Could you check a few things on this drawing? It's one solid part, dimensions in mm from its lowest x, y, z. A direction names the side the tool comes from. Give positions to 0.01 mm unless a question says otherwise; leave off trailing zeros. Loops run counter-clockwise (first coordinate to the right, second up) from the corner with the lowest first, then second, coordinate; pieces in that order, holes last. Notation, with made-up numbers: M 27,75.25 L 79,75.25 A14 ccw 79,94.25 Z; hole C 1.25,46 d7. An arc over 180 degrees is marked long. Answer as CSV lines item,"result". Start each with the question number.
Item 1: For the marked faces 1 and 2, which set-ups out of +Z, -Z, +X, -X, +Y, -Y let a thin tool reach every point of the face, with its end or its side?
Item 2: If I drill on line 1 along Z through (x, y) = (0.95, 52); line 2 along Y through (x, z) = (0.9, 37.4); line 3 along Z through (x, y) = (1.1, 41.5), over which ranges is the centre line in solid material (lowest first)? Write a range as from..to.
Item 3: I want a section at D-D on y = 2.8. List the corners of the cut face in (x, z) for me, plus the area to 3 significant figures.
Item 4: I want a section at B-B on z = 37.4. List the corners of the cut face in (x, y) for me, plus the area to 3 significant figures.
Item 5: I want a section at A-A on y = 30.1. List the corners of the cut face in (x, z) for me, plus the area to 3 significant figures.
Item 6: I want a section at C-C on y = 56. List the corners of the cut face in (x, z) for me.
Item 7: Will these pins go through, and if not, where does the flat tip stop? P1, Ø4.5, axis at y = 2.8, z = 31.1, coming from the -X side; P2, Ø1, axis at x = 1.5, z = 20, coming from the +Y side; P3, Ø1.3, axis at y = 2, z = 16, coming from the -X side; P4, Ø2, axis at y = 30.1, z = 2.8, coming from the +X side.
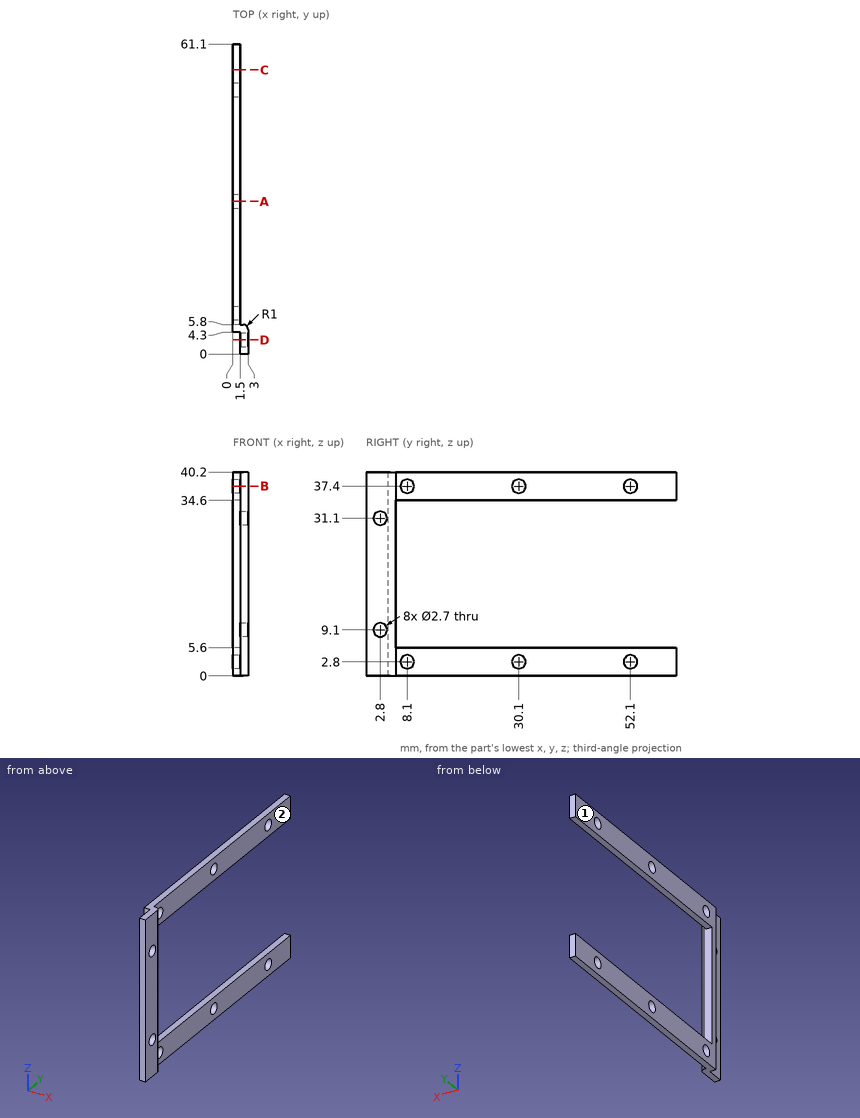
Result:
1,face 1,"+Z, -Z, -X, +Y, -Y"
1,face 2,"+Z, -Z, +X, +Y"
2,line 1,"0..1.45, 4.15..5.6, 34.6..36.05, 38.75..40.2"
2,line 2,"4.3..6.75, 9.45..28.75, 31.45..50.75, 53.45..61.1"
2,line 3,"0..5.6, 34.6..40.2"
3,outline,"M 1.5,0 L 3,0 L 3,7.75 L 1.5,7.75 Z; M 1.5,10.45 L 3,10.45 L 3,29.75 L 1.5,29.75 Z; M 1.5,32.45 L 3,32.45 L 3,40.2 L 1.5,40.2 Z"
3,area,"52.2 mm^2"
4,outline,"M 0,4.3 L 1.5,4.3 L 1.5,0 L 3,0 L 3,4.8 A1 ccw 2,5.8 L 1.5,5.8 L 1.5,6.75 L 0,6.75 Z; M 0,9.45 L 1.5,9.45 L 1.5,28.75 L 0,28.75 Z; M 0,31.45 L 1.5,31.45 L 1.5,50.75 L 0,50.75 Z; M 0,53.45 L 1.5,53.45 L 1.5,61.1 L 0,61.1 Z"
4,area,"81.5 mm^2"
5,outline,"M 0,0 L 1.5,0 L 1.5,1.45 L 0,1.45 Z; M 0,4.15 L 1.5,4.15 L 1.5,5.6 L 0,5.6 Z; M 0,34.6 L 1.5,34.6 L 1.5,36.05 L 0,36.05 Z; M 0,38.75 L 1.5,38.75 L 1.5,40.2 L 0,40.2 Z"
5,area,"8.70 mm^2"
6,outline,"M 0,0 L 1.5,0 L 1.5,5.6 L 0,5.6 Z; M 0,34.6 L 1.5,34.6 L 1.5,40.2 L 0,40.2 Z"
7,P1,"x = 0"
7,P2,"y = 5.8"
7,P3,"x = 1.5"
7,P4,"through"
